```python
from build123d import *

# Parameters (mm, degrees)
F0_R      = 7.5
F0_R_2    = 4
F1_DEPTH  = 22.5
F4_R      = 8
F4_R_2    = 7.15
F5_DEPTH  = 1.1
F6_R      = 8
F6_R_2    = 7.15
F7_DEPTH  = 1.1
F8_R      = 7.15
F8_R_2    = 4.35
F9_DEPTH  = 0.5
F11_R     = 7.15
F11_R_2   = 4.35
F12_DEPTH = 0.5
F13_W     = 1.1570598217
F13_H     = 15.1530206203
F14_DEPTH = 499.5


with BuildPart() as f1:
    # F0 (on Right) → F1 (new body, symmetric)
    with BuildSketch(Plane.YZ):
        Circle(F0_R)
        Circle(F0_R_2, mode=Mode.SUBTRACT)
    extrude(amount=F1_DEPTH, both=True)

    # F4 (on offset) → F5 (cut)
    with BuildSketch(Plane.YZ.offset(-17.5)):
        Circle(F4_R)
        Circle(F4_R_2, mode=Mode.SUBTRACT)
    extrude(amount=F5_DEPTH, mode=Mode.SUBTRACT)

    # F6 (on offset) → F7 (cut)
    with BuildSketch(Plane.YZ.offset(17.5)):
        Circle(F6_R)
        Circle(F6_R_2, mode=Mode.SUBTRACT)
    extrude(amount=-F7_DEPTH, mode=Mode.SUBTRACT)

    # F8 (on face) → F9 (cut)
    with BuildSketch(Plane.YZ.offset(22.5)):
        Circle(F8_R)
        Circle(F8_R_2, mode=Mode.SUBTRACT)
    extrude(amount=-F9_DEPTH, mode=Mode.SUBTRACT)

    # F11 (on face) → F12 (cut)
    with BuildSketch(Plane(origin=(-22.5, 0, 0), x_dir=(0, -1, 0), z_dir=(-1, 0, 0))):
        Circle(F11_R)
        Circle(F11_R_2, mode=Mode.SUBTRACT)
    extrude(amount=-F12_DEPTH, mode=Mode.SUBTRACT)

    # F13 (on face) → F14 (cut, symmetric)
    with BuildSketch(Plane.YZ.offset(22)):
        with Locations((0.8341596586, 7.5765103102)):
            Rectangle(F13_W, F13_H)
    extrude(amount=F14_DEPTH, both=True, mode=Mode.SUBTRACT)


solid = f1.part
```
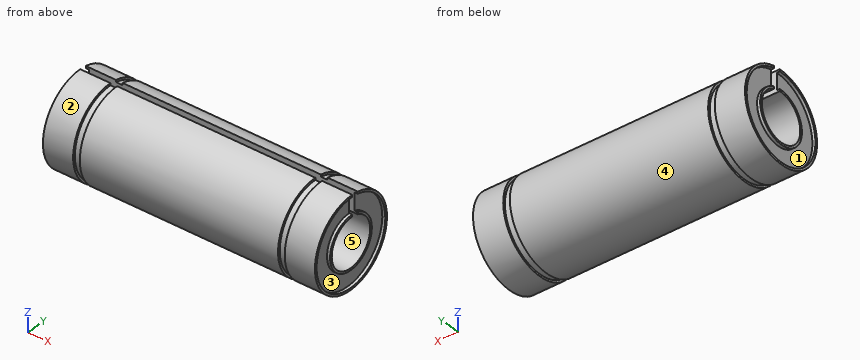
The model under review builds one solid part; all positions refer to its coordinate system, in mm. Face numbers are marked on the shaded views. A direction names the side the tool comes from. Coordinates: 2 decimals unless noted, no trailing zeros. Write each loop counter-clockwise with the first axis right and the second up, starting at its lowest first coordinate (ties: lowest second). Pieces come first, ordered by that corner, then holes.
1) Clearance check with flat-ended pins moving along their axes: pin 1 Ø1.5 at (x, z) = (5.5, -2.5) entering from +Y; pin 2 Ø1.5 at (x, y) = (-15.5, 6) entering from -Z; pin 3 Ø1.5 at (x, z) = (-7.5, 6) entering from -Y. State where each tip first meets the part, or that it passes through.
2) We need section C-C on x = -15. State the section outline as (y, z) points, then the cut area to 3 significant figures.
3) We need section D-D on y = -6. State the section outline as (x, z) points.
4) The part is to be moulded in two halves that separate along Y. For the marked faces 4 and 5, say which applies: pulls with the +Y half, pulls with the -Y half, needs draft (parallel to the pull), parting line crosses it, or undercut.
5) We need section B-B on y = 5.25. State the section outline as (x, z) points.
6) To check wall thickness, follow probe 1 along Y at (x, z) = (22.35, 0); probe 2 along Y at (x, z) = (3, 0). State the ranges of each line that lie inside material, in increasing order.
7) Machinability: for the marked faces 1, 2 and 3, which of the approach directions +Z, -Z, +X, -X, +Y, -Y give a long, thin tool a straight path to every point of the face, cutting with its end or side? Answer none if there is none.
Answer list:
1. pin 1: stops at y = 7.29
1. pin 2: stops at z = -5.36
1. pin 3: stops at y = -5.36
2. outline: (0.26, 3.99) - (0.26, 7.5) arc R7.5 ccw (long way) to (1.41, 7.37) - (1.41, 3.74) arc R4 cw (long way) to start
2. area: 122 mm2
3. outline: (-22.5, -4.5) - (-17.5, -4.5) - (-17.5, -3.89) - (-16.4, -3.89) - (-16.4, -4.5) - (16.4, -4.5) - (16.4, -3.89) - (17.5, -3.89) - (17.5, -4.5) - (22.5, -4.5) - (22.5, -3.89) - (22, -3.89) - (22, 3.89) - (22.5, 3.89) - (22.5, 4.5) - (17.5, 4.5) - (17.5, 3.89) - (16.4, 3.89) - (16.4, 4.5) - (-16.4, 4.5) - (-16.4, 3.89) - (-17.5, 3.89) - (-17.5, 4.5) - (-22.5, 4.5) - (-22.5, 3.89) - (-22, 3.89) - (-22, -3.89) - (-22.5, -3.89) - close
4. face 4: parting line crosses it
4. face 5: undercut
5. outline: (-22.5, -5.36) - (-17.5, -5.36) - (-17.5, -4.85) - (-16.4, -4.85) - (-16.4, -5.36) - (16.4, -5.36) - (16.4, -4.85) - (17.5, -4.85) - (17.5, -5.36) - (22.5, -5.36) - (22.5, -4.85) - (22, -4.85) - (22, 4.85) - (22.5, 4.85) - (22.5, 5.36) - (17.5, 5.36) - (17.5, 4.85) - (16.4, 4.85) - (16.4, 5.36) - (-16.4, 5.36) - (-16.4, 4.85) - (-17.5, 4.85) - (-17.5, 5.36) - (-22.5, 5.36) - (-22.5, 4.85) - (-22, 4.85) - (-22, -4.85) - (-22.5, -4.85) - close
6. probe 1: y = -7.5 to -7.15, -4.35 to -4, 4 to 4.35, 7.15 to 7.5
6. probe 2: y = -7.5 to -4, 4 to 7.5
7. face 1: -X
7. face 2: +X, -X
7. face 3: +X
